Model file for the job. Use its own axes, mm. Face numbers are marked on the shaded views. Coordinates: 2 decimals unless noted, no trailing zeros. Write each loop counter-clockwise with the first axis right and the second up, starting at its lowest first coordinate (ties: lowest second). Pieces come first, ordered by that corner, then holes. Notation, with made-up numbers: M 0,7 L 41,7 A23 ccw 41,41 Z; hole C 35,84.5 d6. An arc over 180 degrees is marked long. Use CSV: the item, a comma, the result in double quotes. Start each with the question number.
from build123d import *

# Parameters (mm, degrees)
SKETCH_1_R            = 15.1
EXTRUDE_1_DEPTH       = 39
SKETCH_4_R            = 11.1
CUT_EXTRUDE_475_DEPTH = 45.463693054
EXTRUDE_START         = -39
SKETCH_1_6_R          = 15.1
EXTRUDE_3_DEPTH       = 39
SKETCH_12_R           = 11
CUT_EXTRUDE_2_DEPTH   = 80


with BuildPart() as part:
    # Sketch 1 → Extrude 1 (new body)
    with BuildSketch(Plane.XY):
        Circle(SKETCH_1_R)
    extrude(amount=EXTRUDE_1_DEPTH)

    # Sketch 4 → Cut-Extrude 475 (cut, through all)
    with BuildSketch(Plane.XY.offset(39)):
        Circle(SKETCH_4_R)
    extrude(amount=-CUT_EXTRUDE_475_DEPTH, mode=Mode.SUBTRACT)

    # Sketch 8 → Cut-Revolve 1 (revolve, cut)
    with BuildSketch(Plane(origin=(0, 0, 0), x_dir=(1, 0, 0), z_dir=(0, 1, 0)), mode=Mode.PRIVATE) as cut_revolve_1_sk:
        Polygon((-11.1, -37), (-11.1, -39), (-13.1, -39), align=None)
    revolve(cut_revolve_1_sk.sketch.rotate(Axis((0, 0, 0), (0, 0, -1)), 180), axis=Axis((0, 0, 0), (0, 0, -1)), mode=Mode.SUBTRACT)

    # Sketch 1_6 → Extrude 3 (add)
    with BuildSketch(Plane.XY.offset(EXTRUDE_START)):
        Circle(SKETCH_1_6_R)
    extrude(amount=EXTRUDE_3_DEPTH)

    # Sketch 12 → Cut-Extrude 2 (cut)
    with BuildSketch(Plane.XY):
        Circle(SKETCH_12_R)
    extrude(amount=-CUT_EXTRUDE_2_DEPTH, mode=Mode.SUBTRACT)

    # Sketch 14 → Cut-Revolve 2 (revolve, cut)
    with BuildSketch(Plane(origin=(0, 0, 0), x_dir=(1, 0, 0), z_dir=(0, 1, 0))):
        Polygon((11, 39), (13, 39), (11, 37), align=None)
    revolve(axis=Axis((0, 0, -39), (0, 0, 1)), mode=Mode.SUBTRACT)


solid = part.part
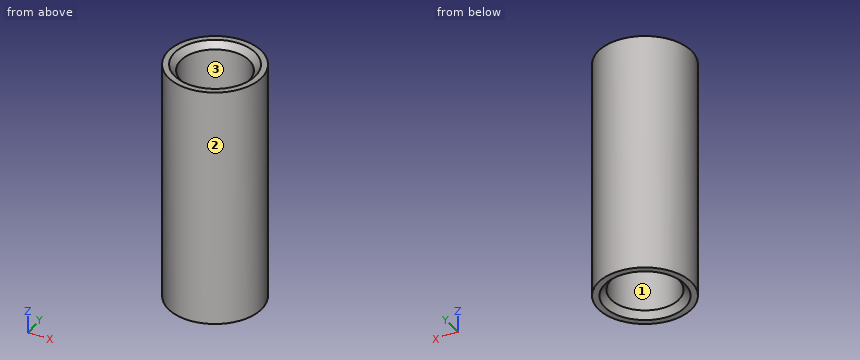
1) Band-saw the part on A-A on x = 0. List the corners of the cut face in (y, z), then the cut area to 3 significant figures.
2) Drop flat-ended pins along their axis: P1, Ø2, axis at x = -3.5, z = 23.5, coming from the -Y side; P2, Ø5, axis at x = 11.5, z = 26, coming from the +Y side; P3, Ø5, axis at x = 10.5, z = -3, coming from the -Y side. Give the stop position or say it passes through.
3) Wall check: L1, parallel to Y at x = 0, z = -25; L2, parallel to Y at x = 0, z = 26; L3, parallel to X at y = -4, z = 14. Give the ranges that are in metal, low to high. Write a range as [from, to].
4) Two-plate mould, pull along Y, no slides. Class the marked faces 1, 2 and 3: pulls with the +Y half, pulls with the -Y half, needs draft (parallel to the pull), parting line crosses it, or undercut.
5) Band-saw the part on C-C on z = 20.5. List the corners of the cut face in (x, y), then the cut area to 3 significant figures.
6) Band-saw the part on D-D on z = -21.5. List the corners of the cut face in (x, y).
Findings below:
1,outline,"M -15.1,-39 L -13,-39 L -11,-37 L -11,0 L -11.1,0 L -11.1,37 L -13.1,39 L -15.1,39 Z; M 11,-37 L 13,-39 L 15.1,-39 L 15.1,39 L 13.1,39 L 11.1,37 L 11.1,0 L 11,0 Z"
1,area,"624 mm2"
2,P1,"stops at y = -14.89"
2,P2,"stops at y = 12.12"
2,P3,"stops at y = -12.81"
3,L1,"y = [-15.1, -11], [11, 15.1]"
3,L2,"y = [-15.1, -11.1], [11.1, 15.1]"
3,L3,"x = [-14.56, -10.35], [10.35, 14.56]"
4,face 1,"undercut"
4,face 2,"parting line crosses it"
4,face 3,"undercut"
5,outline,"C 0,0 d30.2; hole C 0,0 d22.2"
5,area,"329 mm2"
6,outline,"C 0,0 d30.2; hole C 0,0 d22"
